```python
from build123d import *

# Parameters (mm, degrees)
SKETCH1_R           = 50
SKETCH1_R_2         = 35.355339059
BOSS_EXTRUDE1_DEPTH = 69
SKETCH2_R           = 7.911207782
BOSS_EXTRUDE2_DEPTH = 9
CIRPATTERN1_COUNT   = 3


with BuildPart() as part:
    # Sketch1 → Boss-Extrude1 (new body)
    with BuildSketch(Plane(origin=(0, 0, 0), x_dir=(1, 0, 0), z_dir=(0, 1, 0))):
        Circle(SKETCH1_R)
        Circle(SKETCH1_R_2, mode=Mode.SUBTRACT)
    extrude(amount=BOSS_EXTRUDE1_DEPTH)

    # Sketch2 → Boss-Extrude2 (add)
    with BuildSketch(Plane.XZ):
        with BuildLine():
            Line((77.363229747, 12.564610951), (48.395563347, 12.564610951))
            ThreePointArc((48.395563347, 12.564610951), (50, 0), (48.395563347, -12.564610951))
            Line((48.395563347, -12.564610951), (77.363229747, -12.564610951))
            ThreePointArc((77.363229747, -12.564610951), (89.927840698, 0), (77.363229747, 12.564610951))
        make_face()
        with Locations((77.363229747, 0)):
            Circle(SKETCH2_R, mode=Mode.SUBTRACT)
    boss_extrude2 = extrude(amount=-BOSS_EXTRUDE2_DEPTH)

    # CirPattern1: Boss-Extrude2 ×3 about axis
    cirpattern1_axis = Axis((0, 0, 0), (0, 1, 0))
    for i in range(1, CIRPATTERN1_COUNT):
        add(boss_extrude2.rotate(cirpattern1_axis, i * 360 / CIRPATTERN1_COUNT))


solid = part.part
```
Could you check a few things on this model? Use its own coordinates, in mm. A direction names the side the tool comes from. Round coordinates to 2 decimals unless told otherwise and drop trailing zeros. Loops run counter-clockwise (first coordinate to the right, second up) from the corner with the lowest first, then second, coordinate; pieces in that order, holes last.
Q1. On a 3-axis mill with a long thin cutter (end or side, diameter ignored), from which of +Z, -Z, +X, -X, +Y, -Y can I reach the whole of each face in a straight line? I mean faces 1 (the flat face through (-32, 9, 56)), 2 (the flat face through (-32, 9, -56)), 3 (the flat face through (-42.422, 4.437, 48.348)), 4 (the flat face through (63, 4, -12.565)). Say none if no direction works.
Q2. I want a section at D-D (y = 18). Write out the boundary of the cut face in (x, z), and give its area (3 significant figures).
Q3. I want a section at A-A (z = 0). Write out the boundary of the cut face in (x, y).
Q4. I want a section at C-C (z = -21). Write out the boundary of the cut face in (x, y), and give its area (3 significant figures).
Q5. Thinking about a two-plate mould opening in X: for faces 5 (the flat face through (-2, 0, 36)), 6 (the cylindrical face through (33.723, 34.017, -10.62)), 7 (the flat face through (-42.22, 4.44, -48)), which applies, pulls with the +X half, pulls with the -X half, needs draft (parallel to the pull), parting line crosses it, or undercut?
Q6. For P1, Ø3, axis at x = 1.5, y = 12, coming from the -Z side; P2, Ø10, axis at x = -3, y = 49.5, coming from the +Z side; P3, Ø7, axis at x = 63.5, y = 3, coming from the +Z side, each with a flat end and sliding along its axis, tell me the tip position at first contact or that it passes through.
Q7. Please list where these lines run through material, in increasing order: L1, parallel to Z at x = -31.5, y = 4.5; L2, parallel to Z at x = -1, y = 59; L3, parallel to Z at x = -18.5, y = 33.
Q8. I want a section at B-B (x = 0). Write out the boundary of the cut face in (y, z), and give its area (3 significant figures).
Answer below:
1. face 1: +Z, -X, +Y
1. face 2: -Z, -X, +Y
1. face 3: -X, +Y, -Y
1. face 4: -Z, +X, +Y, -Y
2. outline: circle Ø100 at (0, 0); hole circle Ø70.71 at (0, 0)
2. area: 3,930 mm2
3. outline: (-50, 0) - (-35.36, 0) - (-35.36, 69) - (-50, 69) - close; (35.36, 0) - (69.45, 0) - (69.45, 9) - (50, 9) - (50, 69) - (35.36, 69) - close; (85.27, 0) - (89.93, 0) - (89.93, 9) - (85.27, 9) - close
4. outline: (-45.38, 0) - (-28.44, 0) - (-28.44, 69) - (-45.38, 69) - close; (28.44, 0) - (45.38, 0) - (45.38, 69) - (28.44, 69) - close
4. area: 2,340 mm2
5. face 5: needs draft
5. face 6: undercut
5. face 7: pulls with the -X half
6. P1: stops at z = -50
6. P2: stops at z = 50
6. P3: stops at z = 12.56
7. L1: z = -77.31 to -70.32, -63.68 to -16.05, 16.05 to 63.68, 70.32 to 77.31
7. L2: z = -49.99 to -35.34, 35.34 to 49.99
7. L3: z = -46.45 to -30.13, 30.13 to 46.45
8. outline: (0, -50) - (69, -50) - (69, -35.36) - (0, -35.36) - close; (0, 35.36) - (69, 35.36) - (69, 50) - (0, 50) - close
8. area: 2,020 mm2
